from build123d import *
from OCP.BRepFilletAPI import BRepFilletAPI_MakeChamfer

# Parameters (mm, degrees)
BOSS_EXTRUDE1_DEPTH                        = 29.21
SHELL1_T                                   = -2.921
SKETCH3_W                                  = 50.292
SKETCH3_H                                  = 16.1925
CUT_EXTRUDE2_DEPTH                         = 26.9875
BOSS_EXTRUDE2_DEPTH                        = 6.35
FILLET3_R                                  = 1.27
FILLET4_R                                  = 1.27
RIB1_REACH                                 = 116.892
SKETCH6_WALL_W                             = 244.483688888
SKETCH6_WALL_H                             = 2.54
MIRROR2_COPY_1_REACH                       = 116.892
MIRROR2_COPY_1_SKETCH_W                    = 244.483688888
MIRROR2_COPY_1_SKETCH_H                    = 2.54
MIRROR3_COPY_1_REACH                       = 116.892
MIRROR3_COPY_1_SKETCH_W                    = 244.483688888
MIRROR3_COPY_1_SKETCH_H                    = 2.54
MIRROR3_COPY_2_REACH                       = 116.892
MIRROR3_COPY_2_SKETCH_W                    = 244.483688888
MIRROR3_COPY_2_SKETCH_H                    = 2.54
MIRROR3_COPY_3_REACH                       = 116.892
MIRROR3_COPY_3_SKETCH_W                    = 244.483688888
MIRROR3_COPY_3_SKETCH_H                    = 2.54
FILLET6_R                                  = 2.54
SKETCH7_R                                  = 3.3909
CUT_EXTRUDE3_DEPTH                         = 6.35
MIRROR4_AT_THE_SECOND_PLANE_COPY_1_SKETC_R = 3.3909
MIRROR4_AT_THE_SECOND_PLANE_COPY_1_DEPTH   = 6.35
CHAMFER1_SIZE                              = 2.54
CHAMFER1_SIZE2                             = 0.35697372
SKETCH10_W                                 = 17.78
SKETCH10_H                                 = 7.9375
BOSS_EXTRUDE3_DEPTH                        = 2.921
SKETCH11_W                                 = 11.43
SKETCH11_H                                 = 3.175
CUT_EXTRUDE4_DEPTH                         = 2.921
FILLET7_R                                  = 1.5875
FILLET7_OF_MIRROR5_R                       = 1.5875
FILLET8_R                                  = 2.794


with BuildPart() as part:
    # Sketch1 → Boss-Extrude1 (new body)
    with BuildSketch(Plane.XY):
        with BuildLine():
            Line((0, 0), (50.927, 0))
            ThreePointArc((50.927, 0), (59.907256121, 3.719743879), (63.627, 12.7))
            Line((63.627, 12.7), (63.627, 84.1375))
            Line((63.627, 84.1375), (-12.7, 84.1375))
            Line((-12.7, 84.1375), (-12.7, 12.7))
            ThreePointArc((-12.7, 12.7), (-8.980256121, 3.719743879), (0, 0))
        make_face()
    extrude(amount=-BOSS_EXTRUDE1_DEPTH)

    # Shell1
    shell1_openings = [part.faces().sort_by_distance(p)[0] for p in [
        (25.4635, 42.496263873, -29.21),
        (25.4635, 84.1375, -14.605),
    ]]
    offset(amount=SHELL1_T, openings=shell1_openings, kind=Kind.INTERSECTION)

    # Sketch3 → Cut-Extrude2 (cut)
    with BuildSketch(Plane(origin=(0, 0, 0), x_dir=(-1, 0, 0), z_dir=(0, -1, 0))):
        with Locations((-17.2085, 11.27125)):
            Rectangle(SKETCH3_W, SKETCH3_H)
    extrude(amount=-CUT_EXTRUDE2_DEPTH, mode=Mode.SUBTRACT)

    # Sketch4 → Boss-Extrude2 (add)
    with BuildSketch(Plane(origin=(0, 0, -29.21), x_dir=(-1, 0, 0), z_dir=(0, 0, -1))):
        with BuildLine():
            Line((12.7, 17.30375), (19.05, 17.30375))
            ThreePointArc((19.05, 17.30375), (26.67, 24.92375), (19.05, 32.54375))
            Line((19.05, 32.54375), (12.7, 32.54375))
            Line((12.7, 32.54375), (12.7, 17.30375))
        make_face()
        with BuildLine():
            Line((12.7, 79.53375), (19.05, 79.53375))
            ThreePointArc((19.05, 79.53375), (26.67, 71.91375), (19.05, 64.29375))
            Line((19.05, 64.29375), (12.7, 64.29375))
            Line((12.7, 64.29375), (12.7, 79.53375))
        make_face()
        with BuildLine():
            Line((-63.627, 79.53375), (-69.977, 79.53375))
            ThreePointArc((-69.977, 79.53375), (-77.597, 71.91375), (-69.977, 64.29375))
            Line((-69.977, 64.29375), (-63.627, 64.29375))
            Line((-63.627, 64.29375), (-63.627, 79.53375))
        make_face()
        with BuildLine():
            Line((-63.627, 32.54375), (-69.977, 32.54375))
            ThreePointArc((-69.977, 32.54375), (-77.597, 24.92375), (-69.977, 17.30375))
            Line((-69.977, 17.30375), (-63.627, 17.30375))
            Line((-63.627, 17.30375), (-63.627, 32.54375))
        make_face()
    extrude(amount=-BOSS_EXTRUDE2_DEPTH)

    # Fillet3
    fillet3_edges = [part.edges().sort_by_distance(p)[0] for p in [
        (-12.7, 24.92375, -22.86),
        (-12.7, 71.91375, -22.86),
        (63.627, 71.91375, -22.86),
        (63.627, 24.92375, -22.86),
    ]]
    fillet(fillet3_edges, radius=FILLET3_R)

    # Fillet4
    fillet4_edges = [part.edges().sort_by_distance(p)[0] for p in [
        (-7.9375, 4.88712078, -19.3675),
        (42.3545, 1.4605, -3.175),
        (42.3545, 1.4605, -19.3675),
        (-7.9375, 4.88712078, -3.175),
    ]]
    fillet(fillet4_edges, radius=FILLET4_R)

    # Sketch6 wall → Rib1 (add, up to next)
    with BuildSketch(Plane(origin=(66.802, 79.53375, -17.360738686), x_dir=(-0.500000000002, 0, 0.866025403783), z_dir=(0.866025403783, 0, 0.500000000002)), mode=Mode.PRIVATE) as rib1_sk1:
        with Locations((0, 1.27)):
            Rectangle(SKETCH6_WALL_W, SKETCH6_WALL_H)
    rib1_tool1 = extrude(rib1_sk1.sketch, amount=-RIB1_REACH, mode=Mode.PRIVATE) - part.part
    rib1 = rib1_tool1.solids().sort_by_distance((66.802, 79.53375, -17.360738686))[0]
    add(rib1)

    # Mirror1: Rib1 across plane
    add(rib1.mirror(Plane.ZX.offset(71.91375)))

    # Mirror2: Rib1 across plane
    add(rib1.mirror(Plane(origin=(0, 48.41875, 0), x_dir=(0, 0, 1), z_dir=(0, -1, 0))))

    # Mirror2 copy 1 sketch → Mirror2 copy 1 (add, up to next)
    with BuildSketch(Plane(origin=(66.802, 32.54375, -17.360738686), x_dir=(-0.500000000002, 0, 0.866025403783), z_dir=(0.866025403783, 0, 0.500000000002)), mode=Mode.PRIVATE) as mirror2_copy_1_sk1:
        with Locations((0, 1.27)):
            Rectangle(MIRROR2_COPY_1_SKETCH_W, MIRROR2_COPY_1_SKETCH_H)
    mirror2_copy_1_tool1 = extrude(mirror2_copy_1_sk1.sketch, amount=-MIRROR2_COPY_1_REACH, mode=Mode.PRIVATE) - part.part
    add(mirror2_copy_1_tool1.solids().sort_by_distance((66.802, 32.54375, -17.360738686))[0])

    # Mirror3: Rib1 across plane
    add(rib1.mirror(Plane(origin=(25.4635, 0, 0), x_dir=(0, 0, 1), z_dir=(1, 0, 0))))

    # Mirror3 copy 1 sketch → Mirror3 copy 1 (add, up to next)
    with BuildSketch(Plane(origin=(-15.875, 64.29375, -17.360738686), x_dir=(0.500000000002, 0, 0.866025403783), z_dir=(-0.866025403783, 0, 0.500000000002)), mode=Mode.PRIVATE) as mirror3_copy_1_sk1:
        with Locations((0, 1.27)):
            Rectangle(MIRROR3_COPY_1_SKETCH_W, MIRROR3_COPY_1_SKETCH_H)
    mirror3_copy_1_tool1 = extrude(mirror3_copy_1_sk1.sketch, amount=-MIRROR3_COPY_1_REACH, mode=Mode.PRIVATE) - part.part
    add(mirror3_copy_1_tool1.solids().sort_by_distance((-15.875, 64.29375, -17.360738686))[0])

    # Mirror3 copy 2 sketch → Mirror3 copy 2 (add, up to next)
    with BuildSketch(Plane(origin=(-15.875, 17.30375, -17.360738686), x_dir=(0.500000000002, 0, 0.866025403783), z_dir=(-0.866025403783, 0, 0.500000000002)), mode=Mode.PRIVATE) as mirror3_copy_2_sk1:
        with Locations((0, 1.27)):
            Rectangle(MIRROR3_COPY_2_SKETCH_W, MIRROR3_COPY_2_SKETCH_H)
    mirror3_copy_2_tool1 = extrude(mirror3_copy_2_sk1.sketch, amount=-MIRROR3_COPY_2_REACH, mode=Mode.PRIVATE) - part.part
    add(mirror3_copy_2_tool1.solids().sort_by_distance((-15.875, 17.30375, -17.360738686))[0])

    # Mirror3 copy 3 sketch → Mirror3 copy 3 (add, up to next)
    with BuildSketch(Plane(origin=(-15.875, 32.54375, -17.360738686), x_dir=(0.500000000002, 0, 0.866025403783), z_dir=(-0.866025403783, 0, 0.500000000002)), mode=Mode.PRIVATE) as mirror3_copy_3_sk1:
        with Locations((0, -1.27)):
            Rectangle(MIRROR3_COPY_3_SKETCH_W, MIRROR3_COPY_3_SKETCH_H)
    mirror3_copy_3_tool1 = extrude(mirror3_copy_3_sk1.sketch, amount=-MIRROR3_COPY_3_REACH, mode=Mode.PRIVATE) - part.part
    add(mirror3_copy_3_tool1.solids().sort_by_distance((-15.875, 32.54375, -17.360738686))[0])

    # Fillet6
    fillet6_edges = [part.edges().sort_by_distance(p)[0] for p in [
        (-12.7, 17.30375, -20.535738686),
        (-12.7, 32.54375, -20.535738686),
        (-12.7, 64.29375, -20.535738686),
        (-12.7, 79.53375, -20.535738686),
        (63.627, 79.53375, -20.535738686),
        (63.627, 64.29375, -20.535738686),
        (63.627, 32.54375, -20.535738686),
        (63.627, 17.30375, -20.535738686),
    ]]
    fillet(fillet6_edges, radius=FILLET6_R)

    # Sketch7 → Cut-Extrude3 (cut)
    with BuildSketch(Plane.XY.offset(-22.86)):
        with Locations((69.977, 71.91375)):
            Circle(SKETCH7_R)
    cut_extrude3 = extrude(amount=-CUT_EXTRUDE3_DEPTH, mode=Mode.SUBTRACT)

    # Mirror4: Cut-Extrude3 across plane
    add(cut_extrude3.mirror(Plane(origin=(25.4635, 0, 0), x_dir=(0, 0, 1), z_dir=(1, 0, 0))), mode=Mode.SUBTRACT)

    # Mirror4 at the second plane: Cut-Extrude3 across plane
    add(cut_extrude3.mirror(Plane(origin=(0, 48.41875, 0), x_dir=(0, 0, 1), z_dir=(0, -1, 0))), mode=Mode.SUBTRACT)

    # Mirror4 at the second plane copy 1 sketc → Mirror4 at the second plane copy 1 (cut)
    with BuildSketch(Plane(origin=(50.927, 96.8375, -22.86), x_dir=(-1, 0, 0), z_dir=(0, 0, 1))):
        with Locations((69.977, 71.91375)):
            Circle(MIRROR4_AT_THE_SECOND_PLANE_COPY_1_SKETC_R)
    extrude(amount=-MIRROR4_AT_THE_SECOND_PLANE_COPY_1_DEPTH, mode=Mode.SUBTRACT)

    # Chamfer1: one chamfer whose edges measure the first distance from different faces: ONE call of the kernel's chamfer builder (chamfer() names one face for all edges)
    chamfer1_edges_1 = [part.edges().sort_by_distance(p)[0] for p in [
        (66.5861, 71.91375, -29.21),
    ]]
    chamfer1_side_1 = [part.faces().sort_by_distance(p)[0] for p in [
        (66.5861, 71.91375, -26.035),
    ]]
    chamfer1_edges_2 = [part.edges().sort_by_distance(p)[0] for p in [
        (66.5861, 24.92375, -29.21),
    ]]
    chamfer1_side_2 = [part.faces().sort_by_distance(p)[0] for p in [
        (66.5861, 24.92375, -26.035),
    ]]
    chamfer1_edges_3 = [part.edges().sort_by_distance(p)[0] for p in [
        (-15.6591, 71.91375, -29.21),
    ]]
    chamfer1_side_3 = [part.faces().sort_by_distance(p)[0] for p in [
        (-15.6591, 71.91375, -26.035),
    ]]
    chamfer1_edges_4 = [part.edges().sort_by_distance(p)[0] for p in [
        (-15.6591, 24.92375, -29.21),
    ]]
    chamfer1_side_4 = [part.faces().sort_by_distance(p)[0] for p in [
        (-15.6591, 24.92375, -26.035),
    ]]
    chamfer1 = BRepFilletAPI_MakeChamfer(part.part.solid().wrapped)
    for e in chamfer1_edges_1:
        chamfer1.Add(CHAMFER1_SIZE, CHAMFER1_SIZE2, e.wrapped, chamfer1_side_1[0].wrapped)  # the first distance lies on this face
    for e in chamfer1_edges_2:
        chamfer1.Add(CHAMFER1_SIZE, CHAMFER1_SIZE2, e.wrapped, chamfer1_side_2[0].wrapped)  # the first distance lies on this face
    for e in chamfer1_edges_3:
        chamfer1.Add(CHAMFER1_SIZE, CHAMFER1_SIZE2, e.wrapped, chamfer1_side_3[0].wrapped)  # the first distance lies on this face
    for e in chamfer1_edges_4:
        chamfer1.Add(CHAMFER1_SIZE, CHAMFER1_SIZE2, e.wrapped, chamfer1_side_4[0].wrapped)  # the first distance lies on this face
    add(Compound.cast(chamfer1.Shape()), mode=Mode.REPLACE)

    # Sketch10 → Boss-Extrude3 (add)
    with BuildSketch(Plane(origin=(63.627, 0, 0), x_dir=(0, 0, -1), z_dir=(1, 0, 0))):
        with Locations((14.605, 88.10625)):
            Rectangle(SKETCH10_W, SKETCH10_H)
    boss_extrude3 = extrude(amount=-BOSS_EXTRUDE3_DEPTH)

    # Sketch11 → Cut-Extrude4 (cut)
    with BuildSketch(Plane(origin=(63.627, 0, 0), x_dir=(0, 0, -1), z_dir=(1, 0, 0))):
        with Locations((14.605, 87.3125)):
            Rectangle(SKETCH11_W, SKETCH11_H)
    cut_extrude4 = extrude(amount=-CUT_EXTRUDE4_DEPTH, mode=Mode.SUBTRACT)

    # Fillet7
    fillet7_edges = [part.edges().sort_by_distance(p)[0] for p in [
        (62.1665, 85.725, -8.89),
        (62.1665, 88.9, -8.89),
        (62.1665, 88.9, -20.32),
        (62.1665, 85.725, -20.32),
        (62.1665, 92.075, -23.495),
        (62.1665, 92.075, -5.715),
    ]]
    fillet(fillet7_edges, radius=FILLET7_R - 0.0001)  # a hair under: the kernel refuses the full size

    # Mirror5: Boss-Extrude3, Cut-Extrude4 across plane
    add(boss_extrude3.mirror(Plane(origin=(25.4635, 0, 0), x_dir=(0, 0, 1), z_dir=(1, 0, 0))))
    add(cut_extrude4.mirror(Plane(origin=(25.4635, 0, 0), x_dir=(0, 0, 1), z_dir=(1, 0, 0))), mode=Mode.SUBTRACT)

    # Fillet7 of Mirror5
    fillet7_of_mirror5_edges = [part.edges().sort_by_distance(p)[0] for p in [
        (-11.2395, 85.725, -8.89),
        (-11.2395, 88.9, -8.89),
        (-11.2395, 88.9, -20.32),
        (-11.2395, 85.725, -20.32),
        (-11.2395, 92.075, -23.495),
        (-11.2395, 92.075, -5.715),
    ]]
    fillet(fillet7_of_mirror5_edges, radius=FILLET7_OF_MIRROR5_R - 0.0001)  # a hair under: the kernel refuses the full size

    # Fillet8
    fillet8_edges = [part.edges().sort_by_distance(p)[0] for p in [
        (62.1665, 84.1375, -5.715),
        (62.1665, 84.1375, -23.495),
        (-11.2395, 84.1375, -5.715),
        (-11.2395, 84.1375, -23.495),
    ]]
    fillet(fillet8_edges, radius=FILLET8_R)


solid = part.part
Input: part model. Units: mm. Frame: model coordinates. A direction names the side the tool comes from. Coordinates: 2 decimals unless noted, no trailing zeros. Order: outer loops, then holes, each group sorted by start corner. A loop starts at its lowest first (then second) coordinate and runs counter-clockwise, first axis right, second up.
1. Draft query along Y for faces 1 (the cylindrical face through (62.15, 84.93, -4.87)), 2 (the flat face through (68, 64.294, -25)), 3 (the flat face through (-12.7, 53, -11)), 4 (the flat face through (18, 2, -19.368)). Return one class per face: +Y half, -Y half, draft (parallel to the pull), parting line (faces both ways), or undercut.
Checked values:
face 1: +Y half
face 2: undercut
face 3: undercut
face 4: draft
2. Cut plane B-B, the plane y = 56.5. Return loops of the section in (x, z).
Checked values:
outline: (-12.7, -29.21) - (-9.78, -29.21) - (-9.78, -2.92) - (60.71, -2.92) - (60.71, -29.21) - (63.63, -29.21) - (63.63, 0) - (-12.7, 0) - close
3. Cut plane C-C, the plane x = 45.5. Return loops of the section in (y, z).
Checked values:
outline: (0, -29.21) - (2.92, -29.21) - (2.92, -2.92) - (84.14, -2.92) - (84.14, 0) - (0, 0) - close
4. Contact query for flat-ended pins moving along their axis: P1, Ø3, axis at x = 62.5, y = 89.5, coming from the +Z side (3 decimals); P2, Ø4, axis at y = 30, z = -25, coming from the -X side; P3, Ø8, axis at y = 67.5, z = -15.5, coming from the +X side. Output: stop coordinate, or through.
Checked values:
P1: stops at z = -5.715
P2: stops at x = -26.02
P3: stops at x = 68
5. Ray query, line 1 along Y through (x, z) = (-19.05, -24.5); line 2 along X through (y, z) = (70, -4); line 3 along X through (y, z) = (26.5, -23). Return the intervals inside material, ascending.
Checked values:
line 1: y = 17.3 to 21.53, 28.31 to 32.54, 64.29 to 68.52, 75.3 to 79.53
line 2: x = -12.7 to -9.78, 60.71 to 63.63
line 3: x = -26.51 to -22.05, -16.05 to -9.78, 60.71 to 66.97, 72.98 to 77.43
6. Access query for faces 5 (the cylindrical face through (64.39, 63.57, -20.66)), 6 (the flat face through (62, 85.725, -15)), 7 (the cylindrical face through (-13.464, 63.569, -20.414)). Directions: +Z, -Z, +X, -X, +Y, -Y. A direction counts if a zero-diameter tool reaches every point of the face in a straight line with its end or side. Return the directions, or none.
Checked values:
face 5: +Z, -Z, +X
face 6: +X, -X
face 7: +Z, -Z, -X
7. Cut plane D-D, the plane z = -1.75. Return loops of the section in (x, y).
Checked values:
outline: (-12.7, 12.7) arc R12.7 ccw to (0, 0) - (50.93, 0) arc R12.7 ccw to (63.63, 12.7) - (63.63, 84.14) - (-12.7, 84.14) - close
